Autodesk Inventor part; units mm, degrees
ref_plane "YZ Plane" through (0, 0, 0) normal (1, 0, 0) x (0, 1, 0)
ref_plane "XZ Plane" through (0, 0, 0) normal (0, 1, 0) x (-1, 0, 0)
ref_plane "XY Plane" through (0, 0, 0) normal (0, 0, 1) x (1, 0, 0)
sketch "スケッチ1" plane through (0, 0, 0) normal (0, 0, 1) x (1, 0, 0)
  line L0 (-18.25, 14.75) -> (18.25, 14.75)
  line L1 (18.25, 14.75) -> (18.25, -14.75)
  line L2 (18.25, -14.75) -> (-18.25, -14.75)
  line L3 (-18.25, -14.75) -> (-18.25, 14.75)
  line L4 (0, 17.8351) -> (0, -18.1881) construction
  circle A0 centre (0, 7.75) radius 0.5
  circle A1 centre (0, 3.75) radius 0.5
  point P0 (0, 0)
  dimension "d0" = 18.25
  dimension "d1" = 18.25
  dimension "d2" = 14.75
  dimension "d3" = 14.75
  dimension "d18" = 1
  dimension "d19" = 7
  dimension "d20" = 1
  dimension "d21" = 4
extrude "押し出し1" add sketch "スケッチ1" along normal blind 2.25 contours L0 L1 L2 L3 | A0 | A1
sketch "スケッチ2" plane through (0, 0, 2.25) normal (0, 0, 1) x (1, 0, 0)
  line L0 (-17.75, 14.5) -> (17.75, 14.5)
  line L1 (17.75, 14.5) -> (17.75, -14.5)
  line L2 (17.75, -14.5) -> (-17.75, -14.5)
  line L3 (-17.75, -14.5) -> (-17.75, 14.5)
  line L4 (18.25, -14.75) -> (18.25, 14.75)
  point P0 (0, 0)
  dimension "d6" = 0.5
  dimension "d7" = 35.5
  dimension "d8" = 14.5
  dimension "d9" = 14.5
extrude "押し出し2" cut sketch "スケッチ2" against normal blind 0.05
extrude "押し出し5" cut sketch "スケッチ1" along normal blind 1 contours A0 | A1
properties part number "TFT_case"
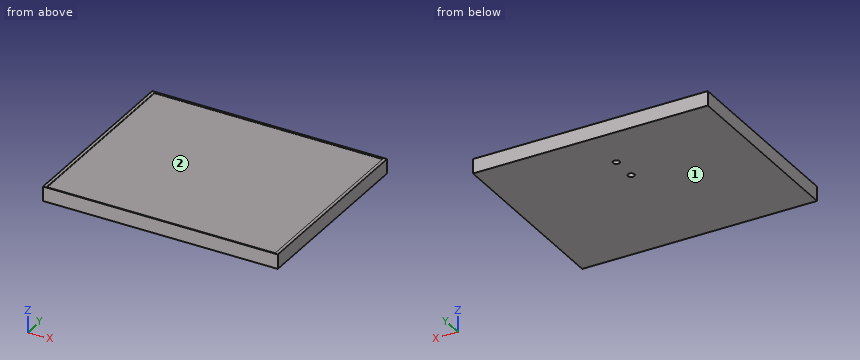
Here's how the part is built. I have some questions about the finished solid (model axes, mm). Face numbers are marked on the shaded views. A direction names the side the tool comes from. Coordinates: 2 decimals unless noted, no trailing zeros. Order: outer loops, then holes, each group sorted by start corner. A loop starts at its lowest first (then second) coordinate and runs counter-clockwise, first axis right, second up. Notation, with made-up numbers: (80, 35.25) - (115, 35.25) arc R19 cw to (115, 52.25) - close; hole circle Ø2 at (-31.75, 35). An arc over 180 degrees is marked (long way). One line per question, with ' | ' between items.
(1) Suppose I cut it at D-D on y = 7.75. List the corners of the cut face in (x, z) for me.
Report:
outline: (-18.25, 0) - (-0.5, 0) - (-0.5, 1) - (0.5, 1) - (0.5, 0) - (18.25, 0) - (18.25, 2.25) - (17.75, 2.25) - (17.75, 2.2) - (-17.75, 2.2) - (-17.75, 2.25) - (-18.25, 2.25) - close
(2) Suppose I cut it at A-A on x = -6. List the corners of the cut face in (y, z) for me, and give its area (3 significant figures).
Report:
outline: (-14.75, 0) - (14.75, 0) - (14.75, 2.25) - (14.5, 2.25) - (14.5, 2.2) - (-14.5, 2.2) - (-14.5, 2.25) - (-14.75, 2.25) - close | area: 64.9 mm2
(3) If I drill on L1, parallel to Y at x = 0, z = 0.65; L2, parallel to Z at x = -6, y = 11.75, over which ranges is the centre line in solid material (lowest first)?
Report:
L1: y = -14.75 to 3.25, 4.25 to 7.25, 8.25 to 14.75 | L2: z = 0 to 2.2
(4) Suppose I cut it at B-B on y = -9.75. List the corners of the cut face in (x, z) for me, and give its area (4 significant figures).
Report:
outline: (-18.25, 0) - (18.25, 0) - (18.25, 2.25) - (17.75, 2.25) - (17.75, 2.2) - (-17.75, 2.2) - (-17.75, 2.25) - (-18.25, 2.25) - close | area: 80.35 mm2
(5) Will this pin go through, and if not, where does the flat tip stop? pin 1 (8.5 mm diameter, centred on x = -1, y = -5, fed in from +Z).
Report:
pin 1: stops at z = 2.2
(6) Suppose I cut it at C-C on x = 0. List the corners of the cut face in (y, z) for me, and give its area (3 significant figures).
Report:
outline: (-14.75, 0) - (3.25, 0) - (3.25, 1) - (4.25, 1) - (4.25, 0) - (7.25, 0) - (7.25, 1) - (8.25, 1) - (8.25, 0) - (14.75, 0) - (14.75, 2.25) - (14.5, 2.25) - (14.5, 2.2) - (-14.5, 2.2) - (-14.5, 2.25) - (-14.75, 2.25) - close | area: 62.9 mm2
(7) For the marked faces 1 and 2, which set-ups out of +Z, -Z, +X, -X, +Y, -Y let a thin tool reach every point of the face, with its end or its side?
Report:
face 1: -Z, +X, -X, +Y, -Y | face 2: +Z
